For this review, take the finished solid that the model builds, in its own axes (mm). Face numbers are marked on the shaded views. A direction names the side the tool comes from. Give positions to 0.01 mm unless a question says otherwise; leave off trailing zeros. Loops run counter-clockwise (first coordinate to the right, second up) from the corner with the lowest first, then second, coordinate; pieces in that order, holes last. Notation, with made-up numbers: (71.25, 80) - (86.25, 80) arc R33 ccw to (86.25, 113) - close; hole circle Ø4 at (75.25, 61.25). An arc over 180 degrees is marked (long way). Answer in a Markdown table with one row per item.
Autodesk Inventor part; units mm, degrees
ref_plane "gn_XY" through (0, 0, 0) normal (0, 0, 1) x (1, 0, 0)
ref_plane "gn_YZ" through (0, 0, 0) normal (1, 0, 0) x (0, 1, 0)
ref_plane "gn_ZX" through (0, 0, 0) normal (0, 1, 0) x (0, 0, 1)
sketch "Sketch_1" plane through (0, 0, 0) normal (0, 0, 1) x (1, 0, 0)
  line L0 (0, -5.5) -> (0, 10.5)
  arc A0 (1, 10.2583) -> (0, 10.9) centre (0, 9.8) ccw
  line L1 (1, 10.2583) -> (1, 10.5)
  line L2 (1, 10.5) -> (2.0574, 10.5)
  line L3 (2.0574, 10.5) -> (2.3025, 10.3151)
  line L4 (2.3025, 10.3151) -> (3.25, 7)
  line L5 (3.25, 7) -> (3.25, 6.5)
  arc A1 (2.5, 4.5) -> (3.25, 6.5) centre (0.0009, 6.5778) ccw
  arc A2 (2.5, 4.5) -> (3.3937, 3) centre (5.3226, 5.1655) ccw
  line L6 (3.3937, 3) -> (5.5, 1.7839)
  line L7 (5.5, 1.7839) -> (5.5, 1.2161)
  line L8 (5.5, 1.2161) -> (3.3937, 0)
  line L9 (3.3937, 0) -> (3.1027, -4.6517)
  line L10 (3.1027, -4.6517) -> (2.1996, -5.5)
  line L11 (2.1996, -5.5) -> (1.3, -5.5)
  line L12 (1.3, -5.5) -> (1.3, -5.1)
  arc A3 (1.3, -5.1) -> (1.7, -4.7) centre (1.3, -4.7) ccw
  line L13 (1.7, -4.7) -> (1.7, 9.55)
  line L14 (1.7, 9.55) -> (1.0067, 10.2433)
  arc A4 (0, 8.7) -> (1.0067, 10.2433) centre (0, 9.8) ccw
  line L15 (0, 8.7) -> (0, 10.9)
revolve "Revolution1" add sketch "Sketch_1" angle 360 about axis through (0, -5.5, 0) along (0, -1, 0)
sketch "Sketch_2" plane through (0, 0, 0) normal (0, 1, 0) x (-1, 0, 0)
  line L0 (6, -6) -> (6, 6)
  line L1 (6, 6) -> (-6, 6)
  line L2 (-6, 6) -> (-6, -6)
  line L3 (-6, -6) -> (6, -6)
  line L4 (3.5, 2.0207) -> (0, 4.0415)
  line L5 (0, 4.0415) -> (-3.5, 2.0207)
  line L6 (-3.5, 2.0207) -> (-3.5, -2.0207)
  line L7 (-3.5, -2.0207) -> (0, -4.0415)
  line L8 (0, -4.0415) -> (3.5, -2.0207)
  line L9 (3.5, -2.0207) -> (3.5, 2.0207)
extrude "Extrusion1" cut sketch "Sketch_2" along normal blind 3
ref_plane "gn_XY" through (0, 0, 0) normal (0, 0, 1) x (1, 0, 0)
ref_plane "gn_YZ" through (0, 0, 0) normal (1, 0, 0) x (0, 1, 0)
ref_plane "gn_ZX" through (0, 0, 0) normal (0, 1, 0) x (0, 0, 1)
properties part number "1/4-28 SAE-LT"
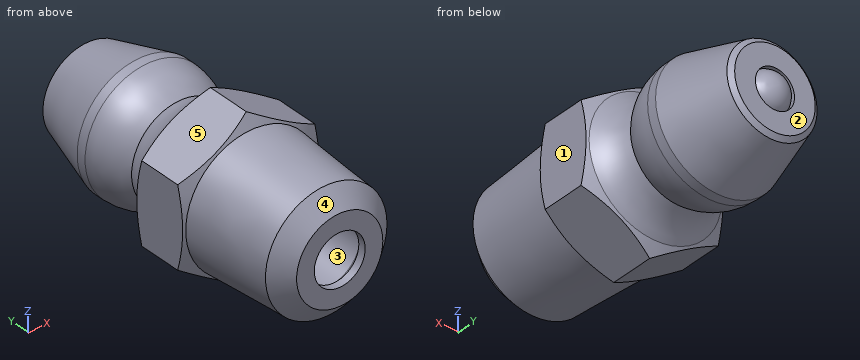
1. Mouldability with a two-part tool opening along X and no side actions: class the marked faces 3, 4 and 5 as released by +X, released by -X, zero draft, split by the parting line, or undercut.
Values:
| item | result |
|---|---|
| face 3 | undercut |
| face 4 | split by the parting line |
| face 5 | released by -X |
2. Clearance check with flat-ended pins moving along their axes: pin 1 (1 mm diameter, centred on x = -1.5, z = 0.5, fed in from +Y); pin 2 (2 mm diameter, centred on x = -1.5, z = -0.5, fed in from +Y); pin 3 (1 mm diameter, centred on y = 5.5, z = 0.5, fed in from -X). State where each tip first meets the part, or that it passes through.
Values:
| item | result |
|---|---|
| pin 1 | stops at y = 10.5 |
| pin 2 | stops at y = 10.73 |
| pin 3 | stops at x = -3.18 |
3. Wall thickness on line 1 (X direction, y = -4, z = -0.5); line 2 (X direction, y = 0.25, z = 1); line 3 (Y direction, x = 1.5, z = 1.25): over which ranges is each line inside the solid? List them lowest first. Write a range as [from, to].
Values:
| item | result |
|---|---|
| line 1 | x = [-3.1, -1.62], [1.62, 3.1] |
| line 2 | x = [-3.5, -1.37], [1.37, 3.5] |
| line 3 | y = [-5.5, 10.5] |
4. We need section A-A, the plane y = -2.5. Give the boundary of the cut face in (x, z).
Values:
| item | result |
|---|---|
| outline | circle Ø6.47 at (0, 0); hole circle Ø3.4 at (0, 0) |
5. We need section B-B, the plane y = 8.5. Give the boundary of the cut face in (x, z), and give its area (3 significant figures).
Values:
| item | result |
|---|---|
| outline | circle Ø5.64 at (0, 0); hole circle Ø3.4 at (0, 0) |
| area | 15.9 mm^2 |
6. For the marked faces 1 and 2, list the 3-axis set-ups (+Z, -Z, +X, -X, +Y, -Y) from which the entire face can be reached by the end or side of a thin tool; tool diameter is ignored.
Values:
| item | result |
|---|---|
| face 1 | +Z, -Z, +X, +Y, -Y |
| face 2 | +Y |
